```python
from build123d import *

# Parameters (mm, degrees)
ESBO_O1_W                = 110
ESBO_O1_H                = 160
RESSALTO_EXTRUS_O1_DEPTH = 3
ESBO_O3_W                = 110
ESBO_O3_H                = 160
ESBO_O3_W_2              = 108
ESBO_O3_H_2              = 158
ESBO_O3_R                = 1
CORTE_EXTRUS_O1_DEPTH    = 98.128780493
ESBO_O5_W                = 87.098953266
ESBO_O5_H                = 10
CORTE_EXTRUS_O2_DEPTH    = 96.739229159
ESBO_O6_W                = 25
ESBO_O6_H                = 5
RESSALTO_EXTRUS_O2_DEPTH = 30
ESBO_O7_W                = 14
ESBO_O7_H                = 20.5
CORTE_EXTRUS_O3_DEPTH    = 171.202820188
ESBO_O8_R                = 1
CORTE_EXTRUS_O4_DEPTH    = 101.284595028
CHANFRO1_SIZE            = 10
FILETE1_R                = 3
FILETE2_R                = 3
CHANFRO2_SIZE            = 1


with BuildPart() as part:
    # Esboço1 → Ressalto-extrusão1 (new body)
    with BuildSketch(Plane(origin=(0, 0, 0), x_dir=(1, 0, 0), z_dir=(0, 1, 0))):
        Rectangle(ESBO_O1_W, ESBO_O1_H)
    extrude(amount=RESSALTO_EXTRUS_O1_DEPTH)

    # Esboço3 → Corte-extrusão1 (cut, through all)
    # profile 1 of 5: a face of its own
    with BuildSketch(Plane(origin=(0, 3, 0), x_dir=(1, 0, 0), z_dir=(0, 1, 0))):
        Rectangle(ESBO_O3_W, ESBO_O3_H)
        Rectangle(ESBO_O3_W_2, ESBO_O3_H_2, mode=Mode.SUBTRACT)
    # profile 2 of 5: a face of its own
    with BuildSketch(Plane(origin=(0, 3, 0), x_dir=(1, 0, 0), z_dir=(0, 1, 0))):
        with Locations(Location((-50, -75, 0), (0, 0, 270))):
            Circle(ESBO_O3_R)
    # profile 3 of 5: a face of its own
    with BuildSketch(Plane(origin=(0, 3, 0), x_dir=(1, 0, 0), z_dir=(0, 1, 0))):
        with Locations(Location((50, -75, 0), (0, 0, 270))):
            Circle(ESBO_O3_R)
    # profile 4 of 5: a face of its own
    with BuildSketch(Plane(origin=(0, 3, 0), x_dir=(1, 0, 0), z_dir=(0, 1, 0))):
        with Locations(Location((50, 75, 0), (0, 0, 270))):
            Circle(ESBO_O3_R)
    # profile 5 of 5: a face of its own
    with BuildSketch(Plane(origin=(0, 3, 0), x_dir=(1, 0, 0), z_dir=(0, 1, 0))):
        with Locations(Location((-50, 75, 0), (0, 0, 270))):
            Circle(ESBO_O3_R)
    extrude(amount=-CORTE_EXTRUS_O1_DEPTH, mode=Mode.SUBTRACT)

    # Esboço5 → Corte-extrusão2 (cut, through all)
    with BuildSketch(Plane(origin=(0, 3, 0), x_dir=(1, 0, 0), z_dir=(0, 1, 0))):
        with Locations((0, 74)):
            Rectangle(ESBO_O5_W, ESBO_O5_H)
    extrude(amount=-CORTE_EXTRUS_O2_DEPTH, mode=Mode.SUBTRACT)

    # Esboço6 → Ressalto-extrusão2 (add)
    with BuildSketch(Plane(origin=(0, 3, 0), x_dir=(1, 0, 0), z_dir=(0, 1, 0))):
        with Locations((26.5, -71.5)):
            Rectangle(ESBO_O6_W, ESBO_O6_H)
    extrude(amount=RESSALTO_EXTRUS_O2_DEPTH)

    # Esboço7 → Corte-extrusão3 (cut, through all)
    with BuildSketch(Plane.XY.offset(79)):
        with Locations((26.5, 16.25)):
            Rectangle(ESBO_O7_W, ESBO_O7_H)
    extrude(amount=-CORTE_EXTRUS_O3_DEPTH, mode=Mode.SUBTRACT)

    # Esboço8 → Corte-extrusão4 (cut, through all)
    with BuildSketch(Plane(origin=(0, 3, 0), x_dir=(1, 0, 0), z_dir=(0, 1, 0))):
        with Locations(Location((-50.46, -54.857726713, 0), (0, 0, 270))):
            Circle(ESBO_O8_R)
        with Locations(Location((-2.2, -56.127726713, 0), (0, 0, 270))):
            Circle(ESBO_O8_R)
        with Locations(Location((-7.28, -4.057726713, 0), (0, 0, 270))):
            Circle(ESBO_O8_R)
        with Locations(Location((-35.22, -4.057726713, 0), (0, 0, 270))):
            Circle(ESBO_O8_R)
        with Locations(Location((48.05, 13.95, 0), (0, 0, 270))):
            Circle(ESBO_O8_R)
        with Locations(Location((2.95, 13.95, 0), (0, 0, 270))):
            Circle(ESBO_O8_R)
        with Locations(Location((-9, 12.482273287, 0), (0, 0, 270))):
            Circle(ESBO_O8_R)
        with Locations(Location((-46, 12.482273287, 0), (0, 0, 270))):
            Circle(ESBO_O8_R)
        with Locations(Location((48.05, 64.05, 0), (0, 0, 270))):
            Circle(ESBO_O8_R)
        with Locations(Location((2.95, 64.05, 0), (0, 0, 270))):
            Circle(ESBO_O8_R)
        with Locations(Location((-9, 65.482273287, 0), (0, 0, 270))):
            Circle(ESBO_O8_R)
        with Locations(Location((-46, 65.482273287, 0), (0, 0, 270))):
            Circle(ESBO_O8_R)
    extrude(amount=-CORTE_EXTRUS_O4_DEPTH, mode=Mode.SUBTRACT)

    # Chanfro1
    # the kernel refuses this chamfer: 10 mm, written as the material it adds along each edge
    with BuildSketch(Plane(origin=(14, 3, 69), x_dir=(0, -0.02749587661058636, -0.9996219169112968), z_dir=(1, 0, 0))) as chanfro1_piece_1_section:
        Polygon((CHANFRO1_SIZE * 0.999621916911, CHANFRO1_SIZE * 0.0274958766106), (-CHANFRO1_SIZE * 0.0274958766106, CHANFRO1_SIZE * 0.999621916911), (0, 0), align=None)
    chanfro1_piece_1 = extrude(amount=25, mode=Mode.PRIVATE)
    chanfro1_piece_1 = split(chanfro1_piece_1, bisect_by=Plane(origin=(16.75, 6, 64.635027274), z_dir=(0, -1, 0)), keep=Keep.TOP, mode=Mode.PRIVATE)
    chanfro1_piece_1 = split(chanfro1_piece_1, bisect_by=Plane(origin=(19.5, 4.275363385, 64.635027274), z_dir=(-1, 0, 0)), keep=Keep.TOP, mode=Mode.PRIVATE)
    add(chanfro1_piece_1)
    with BuildSketch(Plane(origin=(14, 3, 69), x_dir=(0, -0.02749587661058636, -0.9996219169112968), z_dir=(1, 0, 0))) as chanfro1_piece_2_section:
        Polygon((CHANFRO1_SIZE * 0.999621916911, CHANFRO1_SIZE * 0.0274958766106), (-CHANFRO1_SIZE * 0.0274958766106, CHANFRO1_SIZE * 0.999621916911), (0, 0), align=None)
    chanfro1_piece_2 = extrude(amount=25, mode=Mode.PRIVATE)
    chanfro1_piece_2 = split(chanfro1_piece_2, bisect_by=Plane(origin=(16.75, 6, 66.852482787), z_dir=(0, 1, 0)), keep=Keep.TOP, mode=Mode.PRIVATE)
    chanfro1_piece_2 = split(chanfro1_piece_2, bisect_by=Plane(origin=(19.5, 8.478561277, 66.852482787), z_dir=(-1, 0, 0)), keep=Keep.TOP, mode=Mode.PRIVATE)
    add(chanfro1_piece_2)
    with BuildSketch(Plane(origin=(14, 3, 69), x_dir=(0, -0.02749587661058636, -0.9996219169112968), z_dir=(1, 0, 0))) as chanfro1_piece_3_section:
        Polygon((CHANFRO1_SIZE * 0.999621916911, CHANFRO1_SIZE * 0.0274958766106), (-CHANFRO1_SIZE * 0.0274958766106, CHANFRO1_SIZE * 0.999621916911), (0, 0), align=None)
    chanfro1_piece_3 = extrude(amount=25, mode=Mode.PRIVATE)
    chanfro1_piece_3 = split(chanfro1_piece_3, bisect_by=Plane(origin=(33.5, 4.275363385, 64.635027274), z_dir=(-1, 0, 0)), keep=Keep.TOP, mode=Mode.PRIVATE)
    chanfro1_piece_3 = split(chanfro1_piece_3, bisect_by=Plane(origin=(26.5, 6, 64.635027274), z_dir=(0, -1, 0)), keep=Keep.TOP, mode=Mode.PRIVATE)
    chanfro1_piece_3 = split(chanfro1_piece_3, bisect_by=Plane(origin=(19.5, 4.275363385, 64.635027274), z_dir=(1, 0, 0)), keep=Keep.TOP, mode=Mode.PRIVATE)
    add(chanfro1_piece_3)
    with BuildSketch(Plane(origin=(14, 3, 69), x_dir=(0, -0.02749587661058636, -0.9996219169112968), z_dir=(1, 0, 0))) as chanfro1_piece_4_section:
        Polygon((CHANFRO1_SIZE * 0.999621916911, CHANFRO1_SIZE * 0.0274958766106), (-CHANFRO1_SIZE * 0.0274958766106, CHANFRO1_SIZE * 0.999621916911), (0, 0), align=None)
    chanfro1_piece_4 = extrude(amount=25, mode=Mode.PRIVATE)
    chanfro1_piece_4 = split(chanfro1_piece_4, bisect_by=Plane(origin=(33.5, 4.275363385, 64.635027274), z_dir=(1, 0, 0)), keep=Keep.TOP, mode=Mode.PRIVATE)
    chanfro1_piece_4 = split(chanfro1_piece_4, bisect_by=Plane(origin=(36.25, 6, 64.635027274), z_dir=(0, -1, 0)), keep=Keep.TOP, mode=Mode.PRIVATE)
    add(chanfro1_piece_4)
    with BuildSketch(Plane(origin=(14, 3, 69), x_dir=(0, -0.02749587661058636, -0.9996219169112968), z_dir=(1, 0, 0))) as chanfro1_piece_5_section:
        Polygon((CHANFRO1_SIZE * 0.999621916911, CHANFRO1_SIZE * 0.0274958766106), (-CHANFRO1_SIZE * 0.0274958766106, CHANFRO1_SIZE * 0.999621916911), (0, 0), align=None)
    chanfro1_piece_5 = extrude(amount=25, mode=Mode.PRIVATE)
    chanfro1_piece_5 = split(chanfro1_piece_5, bisect_by=Plane(origin=(33.5, 8.478561277, 66.852482787), z_dir=(1, 0, 0)), keep=Keep.TOP, mode=Mode.PRIVATE)
    chanfro1_piece_5 = split(chanfro1_piece_5, bisect_by=Plane(origin=(36.25, 6, 66.852482787), z_dir=(0, 1, 0)), keep=Keep.TOP, mode=Mode.PRIVATE)
    add(chanfro1_piece_5)

    # Filete1
    filete1_edges = [part.edges().sort_by_distance(p)[0] for p in [
        (39, 33, 71.5),
        (14, 33, 71.5),
    ]]
    fillet(filete1_edges, radius=FILETE1_R)

    # Filete2
    filete2_edges = [part.edges().sort_by_distance(p)[0] for p in [
        (-43.549476633, 1.5, -69),
        (43.549476633, 1.5, -69),
    ]]
    fillet(filete2_edges, radius=FILETE2_R)

    # Chanfro2
    chanfro2_edges = [part.edges().sort_by_distance(p)[0] for p in [
        (43.549476633, 3, -75.5),
        (43.549476633, 0, -75.5),
        (0, 3, -69),
        (0, 0, -69),
        (42.670796977, 3, -69.878679656),
        (42.670796977, 0, -69.878679656),
        (-42.670796977, 3, -69.878679656),
        (-42.670796977, 0, -69.878679656),
        (-43.549476633, 0, -75.5),
        (-43.549476633, 3, -75.5),
    ]]
    chamfer(chanfro2_edges, length=CHANFRO2_SIZE)


solid = part.part
```
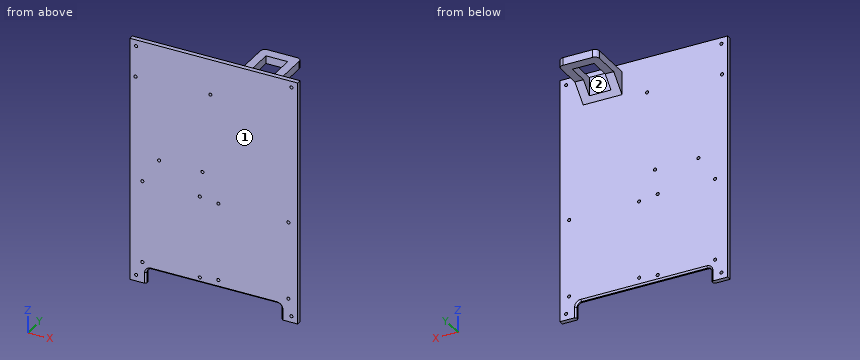
For this review, take the finished solid that the model builds, in its own axes (mm). Face numbers are marked on the shaded views. Give positions to 0.01 mm unless a question says otherwise; leave off trailing zeros. Write each loop counter-clockwise with the first axis right and the second up, starting at its lowest first coordinate (ties: lowest second). Pieces come first, ordered by that corner, then holes. Notation, with made-up numbers: M -38.5,9 L 3.5,9 A22 ccw 3.5,33 Z; hole C 42.25,87 d4. An arc over 180 degrees is marked long. One line per item, written item: value.
1) The part is to be moulded in two halves that separate along Y. For the marked faces 1 and 2, say which applies: +Y half, -Y half, draft (parallel to the pull), parting line (faces both ways), or undercut.
Results are:
face 1: -Y half
face 2: undercut
2) For P1, Ø2.5, axis at x = -7.28, z = 4.06, coming from the +Y side; P2, Ø1.8, axis at x = -46, z = -12.48, coming from the +Y side; P3, Ø4.5, axis at y = 21.5, z = 69.5, coming from the +X side; P4, Ø16.5, axis at y = 20.5, z = 66.5, coming from the -X side, all flat-tipped, find the tip position at first contact; note any pin that passes through.
Results are:
P1: stops at y = 3
P2: passes through
P3: stops at x = 39
P4: stops at x = 14
3) Take a section at D-D, the plane z = -34. Write out the cut boundary in (x, y).
Results are:
outline: M -54,0 L 54,0 L 54,3 L -54,3 Z
4) Take a section at B-B, the plane x = 30.5. Write out the cut boundary in (y, z), then the cut area to 3 significant figures.
Results are:
outline: M 0,-68 L 1,-69 L 2,-69 L 3,-68 L 3,59 L 6,62 L 6,74 L 3,74 L 3,79 L 0,79 Z; M 26.5,69 L 33,69 L 33,74 L 26.5,74 Z
area: 516 mm²
5) Take a section at C-C, the plane x = 12. Write out the cut boundary in (y, z), then the cut area to 3 significant figures.
Results are:
outline: M 0,-68 L 1,-69 L 2,-69 L 3,-68 L 3,79 L 0,79 Z
area: 443 mm²
6) For line 1 (Y direction, x = -2, z = -9); line 2 (Z direction, x = 35.5, y = 31), list the stretches that pass through material, from the lowest coordinate up. Write a range as from..to.
Results are:
line 1: y = 0..3
line 2: z = 69..74
7) Take a section at A-A, the plane y = 21. Write out the cut boundary in (x, z).
Results are:
outline: M 14,69 L 19.5,69 L 19.5,74 L 14,74 Z; M 33.5,69 L 39,69 L 39,74 L 33.5,74 Z
